Source: three-view drawing plus pictorial views. Frame: mm from the lowest corner of the part. Give positions to 0.01 mm unless a question says otherwise; leave off trailing zeros. Loops run counter-clockwise (first coordinate to the right, second up) from the corner with the lowest first, then second, coordinate; pieces in that order, holes last. Notation, with made-up numbers: (51, -24) -> (71, -24) arc R29 cw to (71, 0) -> close; hole circle Ø10 at (-12.75, -2). An arc over 180 degrees is marked (long way). Answer as a JSON object with one key per item and string values. Group by question number.
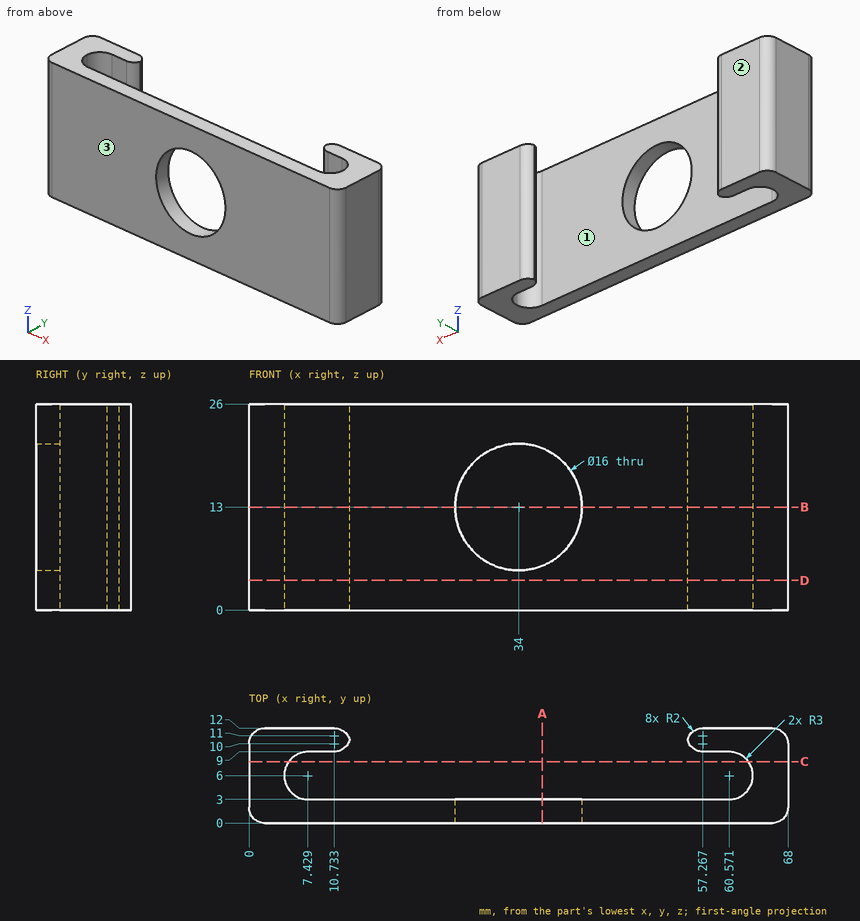
(1) Material intervals for line 1 (Z direction, x = 34, y = 1); line 2 (Y direction, x = 9, z = 13); line 3 (Y direction, x = 22, z = 8.5), sorted ascending. Write a range as from..to.
(2) Section query C-C on y = 7.75. Return the cut outline in (x, z).
(3) Section query B-B on z = 13. Return the cut outline in (x, y).
(4) Mould query, pull axis Y, two halves, no side actions, for the marked faces 1, 2 and 3. Classes: pulls with the +Y half, pulls with the -Y half, needs draft (parallel to the pull), parting line crosses it, or undercut.
(5) Section query D-D on z = 3.75. Return the cut outline in (x, y).
(6) Section query A-A on x = 37. Return the cut outline in (y, z), plus the area to 3 significant figures.
(7) First-contact query: pin 1 (9.5 mm diameter, centred on x = 34, z = 13, fed in from -Y); pin 2 (6 mm diameter, centred on x = 14, z = 14, fed in from +Y); pin 3 (2 mm diameter, centred on x = 40.5, z = 8, fed in from +Y). Flat tips, straight axial feed; report the tip coordinate or a pass-through.
Result:
{
 "1": {"line 1": "0..5, 21..26", "line 2": "0..3, 9..12", "line 3": "0..3"},
 "2": {"outline": "(0, 0) -> (4.99, 0) -> (4.99, 26) -> (0, 26) -> close; (63.01, 0) -> (68, 0) -> (68, 26) -> (63.01, 26) -> close"},
 "3": {"outline": "(0, 2) arc R2 ccw to (2, 0) -> (26, 0) -> (26, 3) -> (7.43, 3) arc R3 cw to (7.43, 9) -> (10.73, 9) arc R2 ccw to (12.67, 10.5) arc R2 ccw to (10.73, 12) -> (2, 12) arc R2 ccw to (0, 10) -> close; (42, 0) -> (66, 0) arc R2 ccw to (68, 2) -> (68, 10) arc R2 ccw to (66, 12) -> (57.27, 12) arc R2 ccw to (55.33, 10.5) arc R2 ccw to (57.27, 9) -> (60.57, 9) arc R3 cw to (60.57, 3) -> (42, 3) -> close"},
 "4": {"face 1": "undercut", "face 2": "pulls with the +Y half", "face 3": "pulls with the -Y half"},
 "5": {"outline": "(0, 2) arc R2 ccw to (2, 0) -> (66, 0) arc R2 ccw to (68, 2) -> (68, 10) arc R2 ccw to (66, 12) -> (57.27, 12) arc R2 ccw to (55.33, 10.5) arc R2 ccw to (57.27, 9) -> (60.57, 9) arc R3 cw to (60.57, 3) -> (7.43, 3) arc R3 cw to (7.43, 9) -> (10.73, 9) arc R2 ccw to (12.67, 10.5) arc R2 ccw to (10.73, 12) -> (2, 12) arc R2 ccw to (0, 10) -> close"},
 "6": {"outline": "(0, 0) -> (3, 0) -> (3, 5.58) -> (0, 5.58) -> close; (0, 20.42) -> (3, 20.42) -> (3, 26) -> (0, 26) -> close", "area": "33.5 mm²"},
 "7": {"pin 1": "through", "pin 2": "y = 11.98", "pin 3": "y = 3"}
}
